Autodesk Inventor part; units mm, degrees
ref_plane "YZ Plane" through (0, 0, 0) normal (1, 0, 0) x (0, 1, 0)
ref_plane "XZ Plane" through (0, 0, 0) normal (0, 1, 0) x (-1, 0, 0)
ref_plane "XY Plane" through (0, 0, 0) normal (0, 0, 1) x (1, 0, 0)
sketch "Esquisse1" plane through (0, 0, 0) normal (0, 1, 0) x (-1, 0, 0)
  circle A0 centre (0, 0) radius 16
  dimension "D" = 32
extrude "Extrusion1" add sketch "Esquisse1" along normal blind 5.5
sketch "Esquisse2" plane through (0, 5.5, 0) normal (0, 1, 0) x (1, 0, 0)
  circle A0 centre (0, 0) radius 16
  circle A1 centre (0, 0) radius 6
  dimension "d3" = 12
extrude "Extrusion2" add sketch "Esquisse2" along normal blind 12 contours A1
sketch "Esquisse4" plane through (0, 17.5, 0) normal (0, 1, 0) x (1, 0, 0)
  circle A0 centre (0, 0) radius 6
  circle A1 centre (0, 0) radius 16
  dimension "d8" = 32
extrude "Extrusion4" add sketch "Esquisse4" along normal blind 2.5 contours A0 | A1
sketch "Esquisse5" plane through (0, 20, 0) normal (0, 1, 0) x (1, 0, 0)
  circle A0 centre (0, 0) radius 16
  circle A1 centre (0, 0) radius 2
  dimension "P" = 4
extrude "Extrusion5" cut sketch "Esquisse5" against normal through all contours A1
sketch "Esquisse6" plane through (0, 0, 0) normal (0, -1, 0) x (1, 0, 0)
  circle A0 centre (0, 0) radius 2
  circle A1 centre (-10, 0) radius 1.5
  circle A2 centre (10, 0) radius 1.5
  dimension "p2" = 3
  dimension "d15" = 3
  dimension "d16" = 20
  dimension "d17" = 10
extrude "Extrusion6" cut sketch "Esquisse6" against normal blind 5.5 contours A1 | A2
sketch "Esquisse7" plane through (0, 20, 0) normal (0, 1, 0) x (1, 0, 0)
  circle A0 centre (0, 0) radius 2
  circle A1 centre (-6.3, 11) radius 1.25
  circle A2 centre (6.3, 11) radius 1.25
  dimension "e" = 2.5
  dimension "d21" = 12.6
  dimension "d22" = 6.3
  dimension "d23" = 11
  dimension "d24" = 2.5
  dimension "d25" = 11
extrude "Extrusion7" cut sketch "Esquisse7" against normal blind 2.5 contours A1 | A2
equation "\"d8\" = D"
equation "\"d15\" = p2"
equation "\"d17\" = 0.5 * d16"
equation "\"d18\" = d1"
equation "\"d22\" = 0.5 * d21"
equation "\"d24\" = e"
equation "\"d25\" = d23"
properties part number "Girouette" material "Plastique ABS"
Could you check a few things on this model? Use its own coordinates, in mm. A direction names the side the tool comes from. Coordinates: 2 decimals unless noted, no trailing zeros. Loops run counter-clockwise (first coordinate to the right, second up) from the corner with the lowest first, then second, coordinate; pieces in that order, holes last.
1) Thinking about a two-plate mould opening in X: for faces 6 (the face through (-5.628, 18.768, -12.054)), 7 (the face through (-6, 11, 0)), 8 (the face through (-7, 5.5, 0)), which applies, released by +X, released by -X, zero draft, split by the parting line, or undercut?
Reported:
face 6: undercut
face 7: split by the parting line
face 8: zero draft
2) Imagine slicing it at B-B (x = 10). List the corners of the cut face in (y, z) for me, and give its area (3 significant figures).
Reported:
outline: (0, -12.49) - (5.5, -12.49) - (5.5, -1.5) - (0, -1.5) - close; (0, 1.5) - (5.5, 1.5) - (5.5, 12.49) - (0, 12.49) - close; (17.5, -12.49) - (20, -12.49) - (20, 12.49) - (17.5, 12.49) - close
area: 183 mm2
3) Please list where these lines run through material, in increasing order: line 1 along Y through (x, z) = (6, 11); line 2 along Z through (x, y) = (0, 9.25); line 3 along Z through (x, y) = (-1.5, 12.5).
Reported:
line 1: y = 0 to 5.5, 17.5 to 20
line 2: z = -6 to -2, 2 to 6
line 3: z = -5.81 to -1.32, 1.32 to 5.81
4) Will these pins go through, and if not, where does the flat tip stop? pin 1 Ø4 at (x, y) = (6.5, 14.5) entering from -Z; pin 2 Ø1.5 at (x, z) = (-6.3, -11) entering from -Y; pin 3 Ø1 at (y, z) = (16, -12) entering from -X; pin 4 Ø8 at (x, y) = (-9, 7) entering from +Z.
Reported:
pin 1: stops at z = -3.97
pin 2: stops at y = 0
pin 3: passes through
pin 4: stops at z = 15.1
5) Imagine slicing it at A-A (x = 0). List the corners of the cut face in (y, z) for me, and give its area (3 significant figures).
Reported:
outline: (0, -16) - (5.5, -16) - (5.5, -6) - (17.5, -6) - (17.5, -16) - (20, -16) - (20, -2) - (0, -2) - close; (0, 2) - (20, 2) - (20, 16) - (17.5, 16) - (17.5, 6) - (5.5, 6) - (5.5, 16) - (0, 16) - close
area: 320 mm2
6) Imagine slicing it at C-C (z = -11). List the corners of the cut face in (x, y) for me.
Reported:
outline: (-11.62, 0) - (11.62, 0) - (11.62, 5.5) - (-11.62, 5.5) - close; (-11.62, 17.5) - (-7.55, 17.5) - (-7.55, 20) - (-11.62, 20) - close; (-5.05, 17.5) - (5.05, 17.5) - (5.05, 20) - (-5.05, 20) - close; (7.55, 17.5) - (11.62, 17.5) - (11.62, 20) - (7.55, 20) - close
7) Imagine slicing it at D-D (y = 12). List the corners of the cut face in (x, z) for me, and give its area (3 significant figures).
Reported:
outline: circle Ø12 at (0, 0); hole circle Ø4 at (0, 0)
area: 101 mm2
8) Which directions (+Z, -Z, +X, -X, +Y, -Y) give clear straight access to the entire face, cutting with the end or side of a thin tool? Please do faces 1 (the face through (0, 20, 3)), 2 (the face through (0, 17.5, 7)), 3 (the face through (0, 0, -3)), 4 (the face through (6.14, 18.77, -12.24)), 5 (the face through (8.5, 2.71, 0.07)).
Reported:
face 1: +Z, -Z, +X, -X, +Y
face 2: none
face 3: +Z, -Z, +X, -X, -Y
face 4: +Y
face 5: -Y
